Could you check a few things on this model? Use its own coordinates, in mm. Give positions to 0.01 mm unless a question says otherwise; leave off trailing zeros. Loops run counter-clockwise (first coordinate to the right, second up) from the corner with the lowest first, then second, coordinate; pieces in that order, holes last. Notation, with made-up numbers: M 17,15 L 50,15 A20 ccw 50,47 Z; hole C -12,31.5 d2. An arc over 180 degrees is marked long. Return JSON: item names as keys, results as strings. Group by question number.
1. If we section it at A-A (y = 149.5): State how many separate pieces and enclosed holes the cut face has, plus the area to 3 significant figures.
2. If we section it at C-C (y = -8): Write out the boundary of the cut face in (x, z), plus the area to 3 significant figures.
3. If we mould it in two halves opening along Y, with no side actions, what happens to faces 1 (the cylindrical face through (1.5, 146.5, -39)), 2 (the flat face through (3, 3, 3))? For each: +Y half, -Y half, draft (parallel to the pull), parting line (faces both ways), or undercut.
4. Please list where these lines run through material, in increasing order: line 1 (Y direction, x = 1.35, z = 43); line 2 (Z direction, x = 1.2, y = 28.5).
5. For pin 1 (0.9 mm diameter, centred on x = 1.5, y = -6.5, fed in from +Z), with a flat end and sliding along its axis, tell me the tip position at first contact or that it passes through.
6. If we section it at B-B (z = 129): Write out the boundary of the cut face in (x, y).
```python
from build123d import *

# Parameters (mm, degrees)
SKETCH_1_W          = 394
SKETCH_1_H          = 399
EXTRUDE_1_DEPTH     = 3
SKETCH_2_R          = 5
SKETCH_2_W          = 7.5
SKETCH_2_H          = 60
CUT_EXTRUDE_1_DEPTH = 281.389461286
FILLET_1_R          = 1


with BuildPart() as part:
    # 草圖1 → 填料-伸長1 (new body)
    with BuildSketch(Plane(origin=(0, 0, 0), x_dir=(0, 0, -1), z_dir=(1, 0, 0))):
        Rectangle(SKETCH_1_W, SKETCH_1_H)
    extrude(amount=EXTRUDE_1_DEPTH)

    # 草圖2 → 除料-伸長1 (cut, through all)
    with BuildSketch(Plane(origin=(3, 0, 0), x_dir=(0, 0, -1), z_dir=(1, 0, 0))):
        with Locations((-129, 149.5)):
            Circle(SKETCH_2_R)
        with Locations((-86, 149.5)):
            Circle(SKETCH_2_R)
        with Locations((-43, 149.5)):
            Circle(SKETCH_2_R)
        with Locations((0, 149.5)):
            Circle(SKETCH_2_R)
        with Locations((43, 149.5)):
            Circle(SKETCH_2_R)
        with Locations((86, 149.5)):
            Circle(SKETCH_2_R)
        with Locations((129, 149.5)):
            Circle(SKETCH_2_R)
        with Locations((-193.25, 0)):
            Rectangle(SKETCH_2_W, SKETCH_2_H)
    extrude(amount=-CUT_EXTRUDE_1_DEPTH, mode=Mode.SUBTRACT)

    # 圓角1
    fillet_1_edges = [part.edges().sort_by_distance(p)[0] for p in [
        (1.5, -30, 197),
        (1.5, 30, 197),
        (1.5, 30, 189.5),
        (1.5, -30, 189.5),
    ]]
    fillet(fillet_1_edges, radius=FILLET_1_R)


solid = part.part
```
Answer:
{
 "1": {"separate pieces": "8", "enclosed holes": "0", "area": "972 mm²"},
 "2": {"outline": "M 0,-197 L 3,-197 L 3,189.5 L 0,189.5 Z", "area": "1,160 mm²"},
 "3": {"face 1": "undercut", "face 2": "draft"},
 "4": {"line 1": "y = -199.5 to 144.5, 154.5 to 199.5", "line 2": "z = -197 to 189.5"},
 "5": {"pin 1": "stops at z = 189.5"},
 "6": {"outline": "M 0,-199.5 L 3,-199.5 L 3,144.5 L 0,144.5 Z; M 0,154.5 L 3,154.5 L 3,199.5 L 0,199.5 Z"}
}
